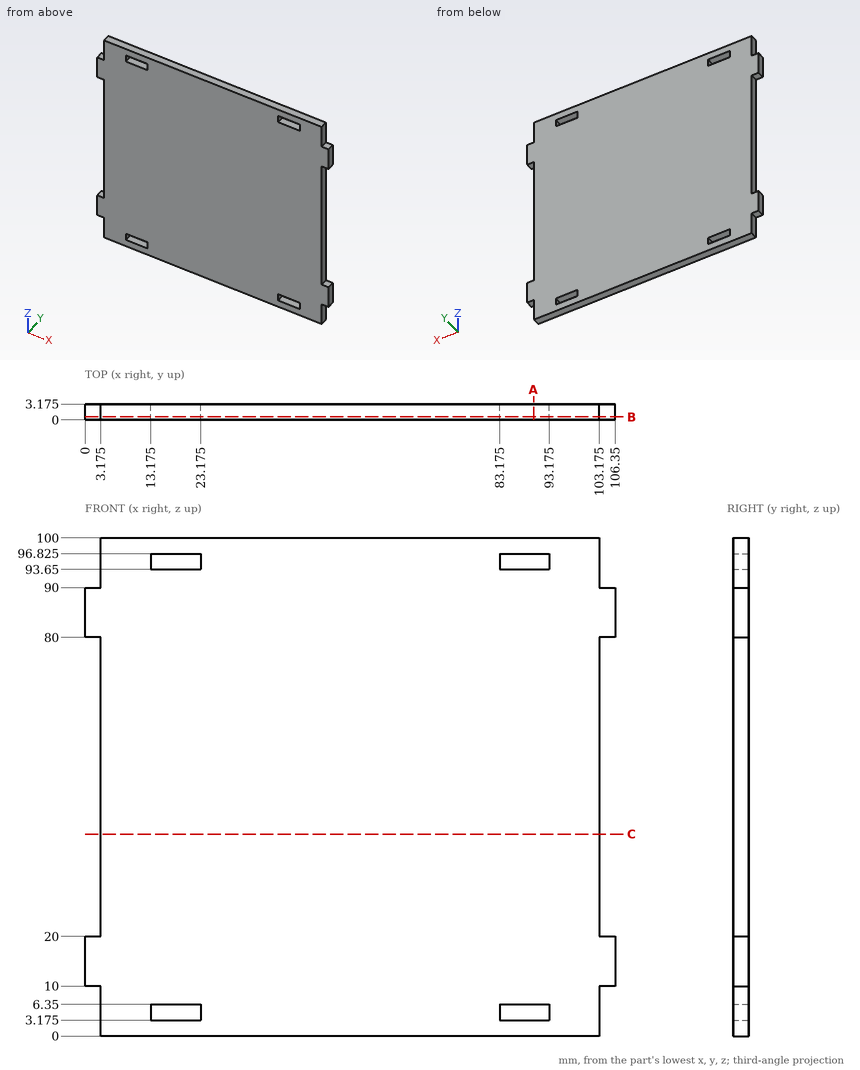
Here's the drawing with two shaded views (mm, measured from the low corner). I have some questions. Coordinates: 2 decimals unless noted, no trailing zeros. Order: outer loops, then holes, each group sorted by start corner. A loop starts at its lowest first (then second) coordinate and runs counter-clockwise, first axis right, second up.
Item 1: I'm going to push flat-ended pins straight in: pin 1 Ø1 at (x, y) = (2, 1) entering from -Z; pin 2 Ø1.5 at (y, z) = (1.5, 54.5) entering from -X (3 decimals); pin 3 Ø6 at (x, z) = (28.5, 26) entering from -Y; pin 4 Ø1.6 at (y, z) = (1, 5.5) entering from +X (3 decimals). Where does each tip first touch, or does it pass through?
Response values:
pin 1: stops at z = 10
pin 2: stops at x = 3.175
pin 3: stops at y = 0
pin 4: stops at x = 103.175
Item 2: I need wall thicknesses on probe 1 along X at (y, z) = (1.6, 4) (3 decimals); probe 2 along Z at (x, y) = (92.5, 2.25) (3 decimals); probe 3 along X at (y, z) = (1.3, 74) (3 decimals). Which ranges of each line are inside material? Lowest first, please.
Response values:
probe 1: x = 3.175 to 13.175, 23.175 to 83.175, 93.175 to 103.175
probe 2: z = 0 to 3.175, 6.35 to 93.65, 96.825 to 100
probe 3: x = 3.175 to 103.175
Item 3: If we section it at C-C, the plane z = 40.5: List the corners of the cut face in (x, y) for me (3 decimals).
Response values:
outline: (3.175, 0) - (103.175, 0) - (103.175, 3.175) - (3.175, 3.175) - close
Item 4: If we section it at A-A, the plane x = 90: List the corners of the cut face in (y, z) for me (3 decimals).
Response values:
outline: (0, 0) - (3.175, 0) - (3.175, 3.175) - (0, 3.175) - close; (0, 6.35) - (3.175, 6.35) - (3.175, 93.65) - (0, 93.65) - close; (0, 96.825) - (3.175, 96.825) - (3.175, 100) - (0, 100) - close
Item 5: If we section it at B-B, the plane y = 0.6: Give the number of separate pieces and of enclosed holes in the cut face, then the cut area to 3 significant figures.
Response values:
separate pieces: 1
enclosed holes: 4
area: 10,000 mm2
